Work out the finished part from the listing and answer in its coordinate system (mm). Coordinates: 2 decimals unless noted, no trailing zeros. Order: outer loops, then holes, each group sorted by start corner. A loop starts at its lowest first (then second) coordinate and runs counter-clockwise, first axis right, second up. Notation, with made-up numbers: M 12,48.25 L 29,48.25 A28 ccw 29,86.25 Z; hole C 41.25,-21.75 d1. An arc over 180 degrees is marked long. Use a Markdown table: item, result.
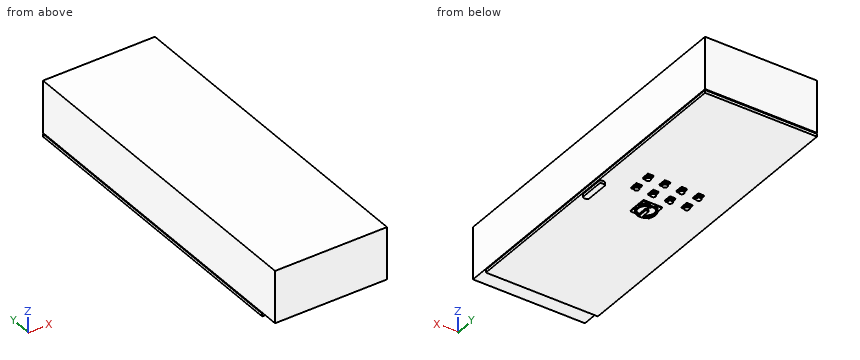
Autodesk Inventor part; units mm, degrees
ref_plane "YZ Plane" through (0, 0, 0) normal (1, 0, 0) x (0, 1, 0)
ref_plane "XZ Plane" through (0, 0, 0) normal (0, 1, 0) x (-1, 0, 0)
ref_plane "XY Plane" through (0, 0, 0) normal (0, 0, 1) x (1, 0, 0)
sketch "Skizze1" plane through (0, 0, 0) normal (0, 1, 0) x (-1, 0, 0)
  line L0 (0, 0) -> (600, 0)
  line L1 (600, 0) -> (600, -280)
  line L2 (600, -280) -> (0, -280)
  line L3 (0, -280) -> (0, 0)
  dimension "d0" = 600
  dimension "d1" = 280
extrude "Extrusion1" add sketch "Skizze1" along normal blind 1800
sketch "Skizze2" plane through (0, 0, -280) normal (0, 0, -1) x (-1, 0, 0)
  line L0 (10, 1790) -> (590, 1790)
  line L1 (590, 1790) -> (590, 110)
  line L2 (590, 110) -> (10, 110)
  line L3 (10, 110) -> (10, 1790)
  line L4 (0, 0) -> (0, 1800)
  line L5 (600, 0) -> (600, 1800)
  line L6 (0, 1800) -> (600, 1800)
  line L7 (0, 0) -> (600, 0)
  dimension "d4" = 10
  dimension "d5" = 10
  dimension "d6" = 10
  dimension "d7" = 110
extrude "Extrusion2" add sketch "Skizze2" along normal blind 5 contours L0 L1 L2 L3
sketch "Skizze3" plane through (0, 0, -285) normal (0, 0, -1) x (-1, 0, 0)
  line L0 (0, 0) -> (0, 1800)
  line L1 (600, 0) -> (600, 1800)
  line L2 (0, 1800) -> (600, 1800)
  line L3 (600, 1800) -> (600, 100)
  line L4 (600, 100) -> (0, 100)
  line L5 (0, 100) -> (0, 1800)
  line L6 (10, 110) -> (590, 110)
  point P0 (0, 100)
  dimension "d10" = 10
extrude "Extrusion3" add sketch "Skizze3" along normal blind 15
sketch "Skizze4" plane through (0, 0, -300) normal (0, 0, -1) x (-1, 0, 0)
  line L0 (15, 980) -> (25, 980)
  line L1 (35, 970) -> (35, 850)
  line L2 (25, 840) -> (15, 840)
  line L3 (5, 850) -> (5, 970)
  line L4 (0, 0) -> (600, 0)
  line L5 (0, 1800) -> (0, 100)
  arc A0 (5, 850) -> (15, 840) centre (15, 850) ccw
  arc A1 (25, 840) -> (35, 850) centre (25, 850) ccw
  arc A2 (35, 970) -> (25, 980) centre (25, 970) ccw
  arc A3 (15, 980) -> (5, 970) centre (15, 970) ccw
  dimension "d13" = 840
  dimension "d14" = 140
  dimension "d15" = 30
  dimension "d16" = 5
  dimension "d17" = 10
extrude "Extrusion4" add sketch "Skizze4" along normal blind 15
sketch "Skizze5" plane through (0, 0, -300) normal (0, 0, -1) x (-1, 0, 0)
  line L0 (150, 1140) -> (180, 1140)
  line L1 (180, 1140) -> (180, 1100)
  line L2 (180, 1100) -> (150, 1100)
  line L3 (150, 1100) -> (150, 1140)
  line L4 (0, 100) -> (600, 100)
  line L5 (0, 1800) -> (0, 100)
  line L6 (240, 1140) -> (270, 1140)
  line L7 (270, 1140) -> (270, 1100)
  line L8 (270, 1100) -> (240, 1100)
  line L9 (240, 1100) -> (240, 1140)
  line L10 (330, 1140) -> (360, 1140)
  line L11 (360, 1140) -> (360, 1100)
  line L12 (360, 1100) -> (330, 1100)
  line L13 (330, 1100) -> (330, 1140)
  line L14 (420, 1140) -> (450, 1140)
  line L15 (450, 1140) -> (450, 1100)
  line L16 (450, 1100) -> (420, 1100)
  line L17 (420, 1100) -> (420, 1140)
  line L18 (150, 1050) -> (180, 1050)
  line L19 (180, 1050) -> (180, 1010)
  line L20 (180, 1010) -> (150, 1010)
  line L21 (150, 1010) -> (150, 1050)
  line L22 (240, 1050) -> (270, 1050)
  line L23 (270, 1050) -> (270, 1010)
  line L24 (270, 1010) -> (240, 1010)
  line L25 (240, 1010) -> (240, 1050)
  line L26 (330, 1050) -> (360, 1050)
  line L27 (360, 1050) -> (360, 1010)
  line L28 (360, 1010) -> (330, 1010)
  line L29 (330, 1010) -> (330, 1050)
  line L30 (420, 1050) -> (450, 1050)
  line L31 (450, 1050) -> (450, 1010)
  line L32 (450, 1010) -> (420, 1010)
  line L33 (420, 1010) -> (420, 1050)
  line L34 (250, 960) -> (350, 960)
  line L35 (350, 960) -> (350, 860)
  line L36 (350, 860) -> (250, 860)
  line L37 (250, 860) -> (250, 960)
  point P0 (0, 0)
  dimension "d20" = 40
  dimension "d21" = 30
  dimension "d22" = 1000
  dimension "d23" = 150
  dimension "d33" = 90
  dimension "d36" = 90
  dimension "d39" = 100
  dimension "d40" = 100
  dimension "d41" = 250
  dimension "d42" = 50
extrude "Extrusion5" add sketch "Skizze5" along normal blind 5
sketch "Skizze6" plane through (0, 0, -305) normal (0, 0, -1) x (-1, 0, 0)
  circle A0 centre (165, 1120) radius 12.5
  line L0 (180, 1140) -> (150, 1140)
  line L1 (180, 1100) -> (180, 1140)
  circle A1 centre (255, 1120) radius 12.5
  circle A2 centre (345, 1120) radius 12.5
  circle A3 centre (435, 1120) radius 12.5
  circle A4 centre (165, 1030) radius 12.5
  circle A5 centre (255, 1030) radius 12.5
  circle A6 centre (345, 1030) radius 12.5
  circle A7 centre (435, 1030) radius 12.5
  circle A8 centre (300, 910) radius 50
  line L2 (350, 860) -> (350, 960)
  line L3 (350, 960) -> (250, 960)
  arc A9 (308, 866.7334) -> (292, 866.7334) centre (300, 910) ccw
  line L4 (292, 915) -> (292, 866.7334)
  line L5 (308, 915) -> (308, 866.7334)
  line L6 (292, 915) -> (300, 923)
  line L7 (292, 915) -> (303.3137, 915) construction
  line L8 (308, 915) -> (300, 923)
  line L9 (308, 915) -> (319.3137, 915) construction
  point P0 (0, 0)
  dimension "d45" = 25
  dimension "d46" = 20
  dimension "d47" = 15
  dimension "d50" = 90
  dimension "d53" = 90
  dimension "d68" = 100
  dimension "d69" = 88
  dimension "d70" = 45
  dimension "d71" = 135
  dimension "d72" = 8
  dimension "d73" = 8
  dimension "d74" = 5
extrude "Extrusion6" add sketch "Skizze6" along normal blind 10 contours A0 | A1 | A2 | A3 | A4 | A5 | A6 | A7 | A8
sketch "Skizze7" plane through (0, 0, -305) normal (0, 0, -1) x (-1, 0, 0)
  line L0 (292, 942) -> (308, 942)
  line L1 (308, 942) -> (308, 930)
  line L2 (308, 930) -> (292, 930)
  line L3 (292, 930) -> (292, 942)
  line L4 (308, 866.7334) -> (308, 915)
  line L5 (292, 915) -> (292, 866.7334)
  point P0 (0, 0)
  point P1 (300, 923)
  dimension "d75" = 7
  dimension "d76" = 12
extrude "Extrusion7" cut sketch "Skizze7" against normal blind 1
equation "\"d5\" = d4"
equation "\"d6\" = d5"
equation "\"d73\" = d72"
properties part number "Schaltschrank2"
(1) Given P1, Ø1.5, axis at x = -345.5, z = -302, coming from the +Y side; P2, Ø16.5, axis at x = -197, z = -290, coming from the -Y side; P3, Ø5.5, axis at y = 1125.5, z = -303.5, coming from the +X side, each flat-ended and moving along its own axis, determine where each tip first touches the part or whether it passes through.
Conclusion:
| item | result |
|---|---|
| P1 | y = 1140 |
| P2 | y = 100 |
| P3 | x = -150 |
(2) Straight lines are drawn through the part: L1, parallel to X at y = 910, z = -307.75; L2, parallel to Y at x = -300, z = -312; L3, parallel to Z at x = -408, y = 524.5. For each, find the intervals that lie inside material, in ascending order.
Conclusion:
| item | result |
|---|---|
| L1 | -350 to -344, -308 to -292, -256 to -250, -35 to -5 |
| L2 | 860 to 923, 954 to 960 |
| L3 | -300 to 0 |
(3) A cutting plane is placed at A-A (y = 301). Determine the outline of the cut face in (x, z).
Conclusion:
| item | result |
|---|---|
| outline | M -600,-300 L 0,-300 L 0,-285 L -10,-285 L -10,-280 L 0,-280 L 0,0 L -600,0 L -600,-280 L -590,-280 L -590,-285 L -600,-285 Z |
(4) A cutting plane is placed at B-B (x = -76.5). Determine the outline of the cut face in (y, z), then the cut area to 3 significant figures.
Conclusion:
| item | result |
|---|---|
| outline | M 0,-280 L 110,-280 L 110,-285 L 100,-285 L 100,-300 L 1800,-300 L 1800,-285 L 1790,-285 L 1790,-280 L 1800,-280 L 1800,0 L 0,0 Z |
| area | 538,000 mm2 |
